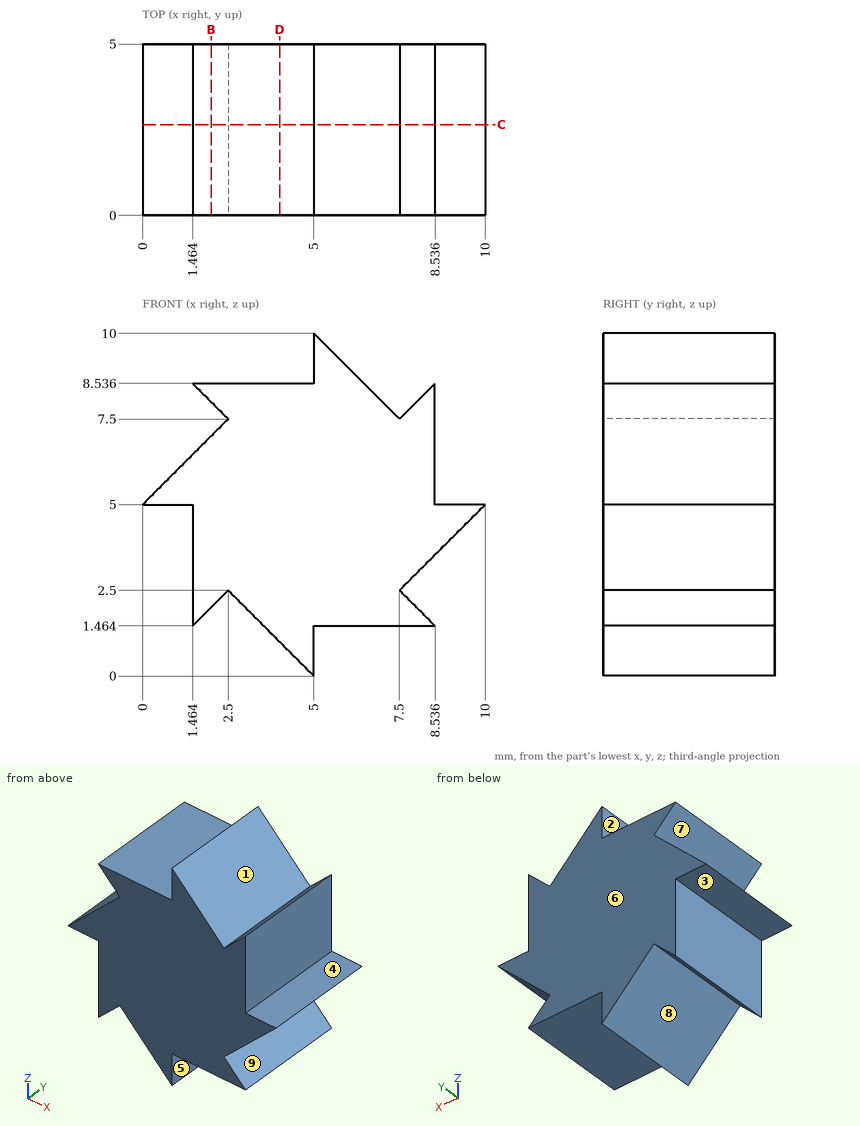
Design review of the part shown in the three views and the two pictorial views. Dimensions are in mm from the part's minimum x, y and z. A direction names the side the tool comes from. Round coordinates to 2 decimals unless told otherwise and drop trailing zeros. Loops run counter-clockwise (first coordinate to the right, second up) from the corner with the lowest first, then second, coordinate; pieces in that order, holes last. Notation, with made-up numbers: (2, -28) -> (9, -28) arc R22 ccw to (9, -12) -> close; hole circle Ø2 at (75, 83). An arc over 180 degrees is marked (long way). Use one line per item in the form item = value. Start each with the question number.
Q1. We need section B-B on x = 2. Give the boundary of the cut face in (y, z) (1 decimal).
Q2. Machinability: for the marked faces 1, 2, 3, 4 and 5, which of the approach directions +Z, -Z, +X, -X, +Y, -Y give a long, thin tool a straight path to every point of the face, cutting with its end or side? Answer none if there is none.
Q3. Wall thickness on line 1 along X through (y, z) = (3.55, 8) (1 decimal); line 2 along Z through (x, y) = (9.75, 2); line 3 along Z through (x, y) = (6, 1.95) (1 decimal): over which ranges is each line inside the solid? List them lowest first. Write a range as [from, to].
Q4. We need section C-C on y = 2.65. Give the boundary of the cut face in (x, z) (1 decimal), then the cut area to 3 significant figures.
Q5. Draft analysis for pull direction Z (two halves, no side actions). For the marked faces 6, 7, 8 and 9, state which applies: +Z half, -Z half, draft (parallel to the pull), parting line (faces both ways), or undercut.
Q6. For pin 1 Ø1.1 at (x, y) = (2.5, 2) entering from +Z; pin 2 Ø1.8 at (y, z) = (1.5, 2.5) entering from -X; pin 3 Ø1.1 at (y, z) = (3, 7) entering from +X, all flat-tipped, find the tip position at first contact; note any pin that passes through.
Q7. We need section D-D on x = 4. Give the boundary of the cut face in (y, z) (1 decimal), then the cut area to 3 significant figures.
Calculated:
q1.outline = (0, 2) -> (5, 2) -> (5, 7) -> (0, 7) -> close; (0, 8) -> (5, 8) -> (5, 8.5) -> (0, 8.5) -> close
q2.face_1 = +Z, +Y, -Y
q2.face_2 = +Z, -X, +Y, -Y
q2.face_3 = -Z, -X, +Y, -Y
q2.face_4 = +Z, +X, +Y, -Y
q2.face_5 = -Z, +X, +Y, -Y
q3.line_1 = [2, 7], [8, 8.5]
q3.line_2 = [4.75, 5]
q3.line_3 = [1.5, 9]
q4.outline = (0, 5) -> (1.5, 5) -> (1.5, 1.5) -> (2.5, 2.5) -> (5, 0) -> (5, 1.5) -> (8.5, 1.5) -> (7.5, 2.5) -> (10, 5) -> (8.5, 5) -> (8.5, 8.5) -> (7.5, 7.5) -> (5, 10) -> (5, 8.5) -> (1.5, 8.5) -> (2.5, 7.5) -> close
q4.area = 50.0 mm²
q5.face_6 = draft
q5.face_7 = undercut
q5.face_8 = -Z half
q5.face_9 = undercut
q6.pin_1 = 8.54
q6.pin_2 = 1.46
q6.pin_3 = 8.54
q7.outline = (0, 1) -> (5, 1) -> (5, 8.5) -> (0, 8.5) -> close
q7.area = 37.7 mm²
